```python
from build123d import *

# Parameters (mm, degrees)
F_01_SQUARE_FLANGE_DEPTH = 6
SKETCH_2_R               = 85
F_02_TUBE_D170_DEPTH     = 100.3
SKETCH_3_R               = 97
F_03_FLANGE_D194_DEPTH   = 6
SKETCH_4_R               = 79
F_04_BORE_D158_DEPTH     = 10
SKETCH_5_R               = 75
F_05_BORE_D150_DEPTH     = 89.3
SKETCH_6_R               = 67
F_06_BORE_D134_DEPTH     = 7
SKETCH_7_R               = 65
F_07_BORE_D130_DEPTH     = 6
SKETCH_8_R               = 2.5
F_08_HOLES_24_D5_DEPTH   = 6
SKETCH_9_R               = 6.75
F_09_HOLES_4_D13_5_DEPTH = 6
SKETCH_10_R              = 1.65
F_10_HOLES_24_M4_DEPTH   = 6


with BuildPart() as part:
    # 草图1 → 01_SQUARE_FLANGE (new body)
    with BuildSketch(Plane.XY):
        Polygon((94.5, 74.5), (94.423893962, 76.243114855), (94.19615506, 77.972963553), (93.818516526, 79.676380902), (93.293852416, 81.340402867), (92.626155741, 82.952365235), (91.820508076, 84.5), (90.883040886, 85.971528727), (89.820888862, 87.355752194), (88.642135624, 88.642135624), (87.355752194, 89.820888862), (85.971528727, 90.883040886), (84.5, 91.820508076), (82.952365235, 92.626155741), (81.340402867, 93.293852416), (79.676380902, 93.818516526), (77.972963553, 94.19615506), (76.243114855, 94.423893962), (74.5, 94.5), (-74.5, 94.5), (-76.243114855, 94.423893962), (-77.972963553, 94.19615506), (-79.676380902, 93.818516526), (-81.340402867, 93.293852416), (-82.952365235, 92.626155741), (-84.5, 91.820508076), (-85.971528727, 90.883040886), (-87.355752194, 89.820888862), (-88.642135624, 88.642135624), (-89.820888862, 87.355752194), (-90.883040886, 85.971528727), (-91.820508076, 84.5), (-92.626155741, 82.952365235), (-93.293852416, 81.340402867), (-93.818516526, 79.676380902), (-94.19615506, 77.972963553), (-94.423893962, 76.243114855), (-94.5, 74.5), (-94.5, -74.5), (-94.423893962, -76.243114855), (-94.19615506, -77.972963553), (-93.818516526, -79.676380902), (-93.293852416, -81.340402867), (-92.626155741, -82.952365235), (-91.820508076, -84.5), (-90.883040886, -85.971528727), (-89.820888862, -87.355752194), (-88.642135624, -88.642135624), (-87.355752194, -89.820888862), (-85.971528727, -90.883040886), (-84.5, -91.820508076), (-82.952365235, -92.626155741), (-81.340402867, -93.293852416), (-79.676380902, -93.818516526), (-77.972963553, -94.19615506), (-76.243114855, -94.423893962), (-74.5, -94.5), (74.5, -94.5), (76.243114855, -94.423893962), (77.972963553, -94.19615506), (79.676380902, -93.818516526), (81.340402867, -93.293852416), (82.952365235, -92.626155741), (84.5, -91.820508076), (85.971528727, -90.883040886), (87.355752194, -89.820888862), (88.642135624, -88.642135624), (89.820888862, -87.355752194), (90.883040886, -85.971528727), (91.820508076, -84.5), (92.626155741, -82.952365235), (93.293852416, -81.340402867), (93.818516526, -79.676380902), (94.19615506, -77.972963553), (94.423893962, -76.243114855), (94.5, -74.5), align=None)
    extrude(amount=F_01_SQUARE_FLANGE_DEPTH)

    # 草图2 → 02_TUBE_D170 (add)
    with BuildSketch(Plane.XY.offset(6)):
        Circle(SKETCH_2_R)
    extrude(amount=F_02_TUBE_D170_DEPTH)

    # 草图3 → 03_FLANGE_D194 (add)
    with BuildSketch(Plane.XY.offset(106.3)):
        Circle(SKETCH_3_R)
    extrude(amount=F_03_FLANGE_D194_DEPTH)

    # 草图4 → 04_BORE_D158 (cut)
    with BuildSketch(Plane.XY):
        Circle(SKETCH_4_R)
    extrude(amount=F_04_BORE_D158_DEPTH, mode=Mode.SUBTRACT)

    # 草图5 → 05_BORE_D150 (cut)
    with BuildSketch(Plane.XY.offset(10)):
        with Locations(Location((0, 0, 0), (0, 0, 180))):
            Circle(SKETCH_5_R)
    extrude(amount=F_05_BORE_D150_DEPTH, mode=Mode.SUBTRACT)

    # 草图6 → 06_BORE_D134 (cut)
    with BuildSketch(Plane.XY.offset(99.3)):
        Circle(SKETCH_6_R)
    extrude(amount=F_06_BORE_D134_DEPTH, mode=Mode.SUBTRACT)

    # 草图7 → 07_BORE_D130 (cut)
    with BuildSketch(Plane.XY.offset(106.3)):
        Circle(SKETCH_7_R)
    extrude(amount=F_07_BORE_D130_DEPTH, mode=Mode.SUBTRACT)

    # 草图8 → 08_HOLES_24_D5 (cut)
    with BuildSketch(Plane.XY.offset(106.3)):
        with Locations((91, 0)):
            Circle(SKETCH_8_R)
        with Locations((87.899250192, 23.552533104)):
            Circle(SKETCH_8_R)
        with Locations((78.808311744, 45.5)):
            Circle(SKETCH_8_R)
        with Locations((64.346717088, 64.346717088)):
            Circle(SKETCH_8_R)
        with Locations((45.5, 78.808311744)):
            Circle(SKETCH_8_R)
        with Locations((23.552533104, 87.899250192)):
            Circle(SKETCH_8_R)
        with Locations((0, 91)):
            Circle(SKETCH_8_R)
        with Locations((-23.552533104, 87.899250192)):
            Circle(SKETCH_8_R)
        with Locations((-45.5, 78.808311744)):
            Circle(SKETCH_8_R)
        with Locations((-64.346717088, 64.346717088)):
            Circle(SKETCH_8_R)
        with Locations((-78.808311744, 45.5)):
            Circle(SKETCH_8_R)
        with Locations((-87.899250192, 23.552533104)):
            Circle(SKETCH_8_R)
        with Locations((-91, 0)):
            Circle(SKETCH_8_R)
        with Locations((-87.899250192, -23.552533104)):
            Circle(SKETCH_8_R)
        with Locations((-78.808311744, -45.5)):
            Circle(SKETCH_8_R)
        with Locations((-64.346717088, -64.346717088)):
            Circle(SKETCH_8_R)
        with Locations((-45.5, -78.808311744)):
            Circle(SKETCH_8_R)
        with Locations((-23.552533104, -87.899250192)):
            Circle(SKETCH_8_R)
        with Locations((0, -91)):
            Circle(SKETCH_8_R)
        with Locations((23.552533104, -87.899250192)):
            Circle(SKETCH_8_R)
        with Locations((45.5, -78.808311744)):
            Circle(SKETCH_8_R)
        with Locations((64.346717088, -64.346717088)):
            Circle(SKETCH_8_R)
        with Locations((78.808311744, -45.5)):
            Circle(SKETCH_8_R)
        with Locations((87.899250192, -23.552533104)):
            Circle(SKETCH_8_R)
    extrude(amount=F_08_HOLES_24_D5_DEPTH, mode=Mode.SUBTRACT)

    # 草图9 → 09_HOLES_4_D13.5 (cut)
    with BuildSketch(Plane.XY):
        with Locations((-65, -65)):
            Circle(SKETCH_9_R)
        with Locations((-65, 65)):
            Circle(SKETCH_9_R)
        with Locations((65, -65)):
            Circle(SKETCH_9_R)
        with Locations((65, 65)):
            Circle(SKETCH_9_R)
    extrude(amount=F_09_HOLES_4_D13_5_DEPTH, mode=Mode.SUBTRACT)

    # 草图10 → 10_HOLES_24_M4 (cut)
    with BuildSketch(Plane.XY.offset(106.3)):
        with Locations((69.401140296, 9.136833455)):
            Circle(SKETCH_10_R)
        with Locations((64.671567276, 26.787840266)):
            Circle(SKETCH_10_R)
        with Locations((55.53473382, 42.613300031)):
            Circle(SKETCH_10_R)
        with Locations((42.613300031, 55.53473382)):
            Circle(SKETCH_10_R)
        with Locations((26.787840266, 64.671567276)):
            Circle(SKETCH_10_R)
        with Locations((9.136833455, 69.401140296)):
            Circle(SKETCH_10_R)
        with Locations((-9.136833455, 69.401140296)):
            Circle(SKETCH_10_R)
        with Locations((-26.787840266, 64.671567276)):
            Circle(SKETCH_10_R)
        with Locations((-42.613300031, 55.53473382)):
            Circle(SKETCH_10_R)
        with Locations((-55.53473382, 42.613300031)):
            Circle(SKETCH_10_R)
        with Locations((-64.671567276, 26.787840266)):
            Circle(SKETCH_10_R)
        with Locations((-69.401140296, 9.136833455)):
            Circle(SKETCH_10_R)
        with Locations((-69.401140296, -9.136833455)):
            Circle(SKETCH_10_R)
        with Locations((-64.671567276, -26.787840266)):
            Circle(SKETCH_10_R)
        with Locations((-55.53473382, -42.613300031)):
            Circle(SKETCH_10_R)
        with Locations((-42.613300031, -55.53473382)):
            Circle(SKETCH_10_R)
        with Locations((-26.787840266, -64.671567276)):
            Circle(SKETCH_10_R)
        with Locations((-9.136833455, -69.401140296)):
            Circle(SKETCH_10_R)
        with Locations((9.136833455, -69.401140296)):
            Circle(SKETCH_10_R)
        with Locations((26.787840266, -64.671567276)):
            Circle(SKETCH_10_R)
        with Locations((42.613300031, -55.53473382)):
            Circle(SKETCH_10_R)
        with Locations((55.53473382, -42.613300031)):
            Circle(SKETCH_10_R)
        with Locations((64.671567276, -26.787840266)):
            Circle(SKETCH_10_R)
        with Locations((69.401140296, -9.136833455)):
            Circle(SKETCH_10_R)
    extrude(amount=F_10_HOLES_24_M4_DEPTH, mode=Mode.SUBTRACT)


solid = part.part
```
CAD build for the part. Positions are in the model's coordinates, mm. A direction names the side the tool comes from. Coordinates: 2 decimals unless noted, no trailing zeros. Write each loop counter-clockwise with the first axis right and the second up, starting at its lowest first coordinate (ties: lowest second). Pieces come first, ordered by that corner, then holes.
(1) 3-axis set-ups, long thin cutter, end or side, ignore diameter. For faces 4 (the face through (62, 19.52, 109.26)), 5 (the face through (0, 87, 106.3)), 6 (the face through (81.193, 46.251, 109.258)), 7 (the face through (-69.975, -60.438, 2.958)): which of +Z, -Z, +X, -X, +Y, -Y reach the whole face in a straight line?
(2) Cut at B-B, the plane z = 25. List the corners of the cut face in (x, y).
(3) Drill centre lines: probe 1 along Z at (x, y) = (-49.5, -70.5); probe 2 along Z at (x, y) = (70, 19.5); probe 3 along Y at (x, z) = (-18.5, 35.5). Where is each one in solid material? Low to high.
(4) Flat gauge pins, fed straight in: pin 1 (4.5 mm diameter, centred on x = -23.55, y = 87.9, fed in from -Z); pin 2 (4 mm diameter, centred on x = -26.79, y = 64.67, fed in from -Z); pin 3 (8 mm diameter, centred on x = -65, y = -65, fed in from -Z); pin 4 (1 mm diameter, centred on y = 40, z = 61.5, fed in from +X). Where does each tip first touch, or does it go through?
(5) Cut at C-C, the plane x = 31. List the corners of the cut face in (y, z), and give its area (3 significant figures).
(6) Cut at A-A, the plane y = 0. Count the separate pieces of the cut face and the enclosed holes in it, and give its area (3 significant figures).
(7) Two-plate mould, pull along X, no slides. Class faces 1 (the face through (-67.453, -51.721, 55.448)), 2 (the face through (94.5, -1, 3)), 3 (the face through (-85.515, -22.802, 109.258)): +X half, -X half, draft (parallel to the pull), parting line (faces both ways), or undercut.
Geometry says:
1. face 4: +Z, -Z
1. face 5: none
1. face 6: +Z
1. face 7: -Z
2. outline: circle Ø170 at (0, 0); hole circle Ø150 at (0, 0)
3. probe 1: z = 0 to 6, 106.3 to 112.3
3. probe 2: z = 99.3 to 112.3
3. probe 3: y = -82.96 to -72.68, 72.68 to 82.96
4. pin 1: stops at z = 0
4. pin 2: stops at z = 99.3
4. pin 3: stops at z = 106.3
4. pin 4: stops at x = 75.26
5. outline: (-94.5, 0) - (-72.66, 0) - (-72.66, 10) - (-68.29, 10) - (-68.29, 99.3) - (-59.4, 99.3) - (-59.4, 106.3) - (-57.13, 106.3) - (-57.13, 112.3) - (-91.91, 112.3) - (-91.91, 106.3) - (-79.15, 106.3) - (-79.15, 6) - (-94.5, 6) - close; (57.13, 106.3) - (59.4, 106.3) - (59.4, 99.3) - (68.29, 99.3) - (68.29, 10) - (72.66, 10) - (72.66, 0) - (94.5, 0) - (94.5, 6) - (79.15, 6) - (79.15, 106.3) - (91.91, 106.3) - (91.91, 112.3) - (57.13, 112.3) - close
5. area: 2,950 mm2
6. separate pieces: 4
6. enclosed holes: 0
6. area: 2,600 mm2
7. face 1: parting line
7. face 2: +X half
7. face 3: undercut
